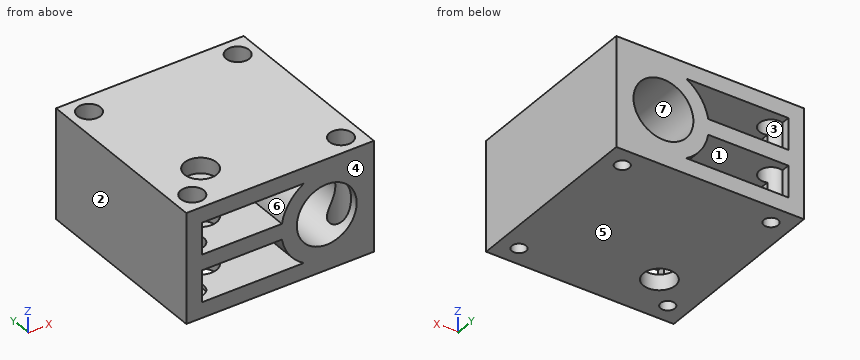
```python
from build123d import *

# Parameters (mm, degrees)
F2_W     = 48.25
F2_H     = 28.25
F2_R     = 7.7
F3_DEPTH = 24.2
F5_R     = 2.975
F6_DEPTH = 25.25
F4_R     = 1.825
F7_DEPTH = 28.25
F4_R_2   = 4.125
F8_DEPTH = 28.25


# Not quite as in the source:
# - a feature names something its author has since deleted; it is built from what else it names


with BuildPart() as f3:
    # F2 (on Front) → F3 (new body, symmetric)
    with BuildSketch(Plane.XZ):
        Rectangle(F2_W, F2_H)
        with BuildLine():
            ThreePointArc((23.5277925033, 2), (23.6568686252, 1.0037000824), (23.7, 0))
            ThreePointArc((23.7, 0), (23.6568686252, -1.0037000824), (23.5277925033, -2))
            ThreePointArc((23.5277925033, -2), (22.3372126342, -5.4801491728), (20.125, -8.4186920005))
            Line((20.125, -8.4186920005), (20.125, -10.125))
            Line((20.125, -10.125), (17.8629663994, -10.125))
            ThreePointArc((17.8629663994, -10.125), (15.9935594213, -10.9973398215), (14, -11.5277925033))
            ThreePointArc((14, -11.5277925033), (12, -11.7), (10, -11.5277925033))
            ThreePointArc((10, -11.5277925033), (8.0064405787, -10.9973398215), (6.1370336006, -10.125))
            Line((6.1370336006, -10.125), (-20.125, -10.125))
            Line((-20.125, -10.125), (-20.125, -2))
            Line((-20.125, -2), (-20.125, 2))
            Line((-20.125, 2), (-20.125, 10.125))
            Line((-20.125, 10.125), (6.1370336006, 10.125))
            ThreePointArc((6.1370336006, 10.125), (8.0064405787, 10.9973398215), (10, 11.5277925033))
            ThreePointArc((10, 11.5277925033), (12, 11.7), (14, 11.5277925033))
            ThreePointArc((14, 11.5277925033), (15.9935594213, 10.9973398215), (17.8629663994, 10.125))
            Line((17.8629663994, 10.125), (20.125, 10.125))
            Line((20.125, 10.125), (20.125, 8.4186920005))
            ThreePointArc((20.125, 8.4186920005), (22.3372126342, 5.4801491728), (23.5277925033, 2))
        make_face(mode=Mode.SUBTRACT)
        with BuildLine():
            Line((14, 10.125), (14, 11.5277925033))
            ThreePointArc((14, 11.5277925033), (12, 11.7), (10, 11.5277925033))
            Line((10, 11.5277925033), (10, 10.125))
            Line((10, 10.125), (14, 10.125))
        make_face()
        with BuildLine():
            Line((20.125, 2), (20.125, 8.4186920005))
            ThreePointArc((20.125, 8.4186920005), (19.045826619, 9.3405742466), (17.8629663994, 10.125))
            Line((17.8629663994, 10.125), (14, 10.125))
            Line((14, 10.125), (10, 10.125))
            Line((10, 10.125), (6.1370336006, 10.125))
            ThreePointArc((6.1370336006, 10.125), (2.4024206149, 6.6915222444), (0.4722074967, 2))
            ThreePointArc((0.4722074967, 2), (0.3, 0), (0.4722074967, -2))
            ThreePointArc((0.4722074967, -2), (2.4024206149, -6.6915222444), (6.1370336006, -10.125))
            Line((6.1370336006, -10.125), (10, -10.125))
            Line((10, -10.125), (14, -10.125))
            Line((14, -10.125), (17.8629663994, -10.125))
            ThreePointArc((17.8629663994, -10.125), (19.045826619, -9.3405742466), (20.125, -8.4186920005))
            Line((20.125, -8.4186920005), (20.125, -2))
            Line((20.125, -2), (20.125, 2))
        make_face()
        with Locations((12, 0)):
            Circle(F2_R, mode=Mode.SUBTRACT)
        with BuildLine():
            ThreePointArc((10, -11.5277925033), (12, -11.7), (14, -11.5277925033))
            Line((14, -11.5277925033), (14, -10.125))
            Line((14, -10.125), (10, -10.125))
            Line((10, -10.125), (10, -11.5277925033))
        make_face()
        with BuildLine():
            ThreePointArc((0.4722074967, -2), (0.3, 0), (0.4722074967, 2))
            Line((0.4722074967, 2), (-20.125, 2))
            Line((-20.125, 2), (-20.125, -2))
            Line((-20.125, -2), (0.4722074967, -2))
        make_face()
        with BuildLine():
            ThreePointArc((23.5277925033, -2), (23.6568686252, -1.0037000824), (23.7, 0))
            ThreePointArc((23.7, 0), (23.6568686252, 1.0037000824), (23.5277925033, 2))
            Line((23.5277925033, 2), (20.125, 2))
            Line((20.125, 2), (20.125, -2))
            Line((20.125, -2), (23.5277925033, -2))
        make_face()
        with BuildLine():
            Line((20.125, 2), (23.5277925033, 2))
            ThreePointArc((23.5277925033, 2), (22.3372126342, 5.4801491728), (20.125, 8.4186920005))
            Line((20.125, 8.4186920005), (20.125, 2))
        make_face()
        with BuildLine():
            ThreePointArc((20.125, -8.4186920005), (22.3372126342, -5.4801491728), (23.5277925033, -2))
            Line((23.5277925033, -2), (20.125, -2))
            Line((20.125, -2), (20.125, -8.4186920005))
        make_face()
        with BuildLine():
            Line((14, 10.125), (17.8629663994, 10.125))
            ThreePointArc((17.8629663994, 10.125), (15.9935594213, 10.9973398215), (14, 11.5277925033))
            Line((14, 11.5277925033), (14, 10.125))
        make_face()
        with BuildLine():
            Line((10, 10.125), (10, 11.5277925033))
            ThreePointArc((10, 11.5277925033), (8.0064405787, 10.9973398215), (6.1370336006, 10.125))
            Line((6.1370336006, 10.125), (10, 10.125))
        make_face()
        with BuildLine():
            ThreePointArc((14, -11.5277925033), (15.9935594213, -10.9973398215), (17.8629663994, -10.125))
            Line((17.8629663994, -10.125), (14, -10.125))
            Line((14, -10.125), (14, -11.5277925033))
        make_face()
        with BuildLine():
            ThreePointArc((6.1370336006, -10.125), (8.0064405787, -10.9973398215), (10, -11.5277925033))
            Line((10, -11.5277925033), (10, -10.125))
            Line((10, -10.125), (6.1370336006, -10.125))
        make_face()
        with BuildLine():
            ThreePointArc((17.8629663994, 10.125), (19.045826619, 9.3405742466), (20.125, 8.4186920005))
            Line((20.125, 8.4186920005), (20.125, 10.125))
            Line((20.125, 10.125), (17.8629663994, 10.125))
        make_face()
        with BuildLine():
            Line((20.125, -10.125), (20.125, -8.4186920005))
            ThreePointArc((20.125, -8.4186920005), (19.045826619, -9.3405742466), (17.8629663994, -10.125))
            Line((17.8629663994, -10.125), (20.125, -10.125))
        make_face()
    extrude(amount=F3_DEPTH, both=True)

    # F5 (on face) → F6 (cut)
    with BuildSketch(Plane.XY.offset(14.125)):
        with Locations((-19.125, 19.2)):
            Circle(F5_R)
        with Locations((19.125, -19.2)):
            Circle(F5_R)
        with Locations((-19.125, -19.2)):
            Circle(F5_R)
        with Locations((19.125, 19.2)):
            Circle(F5_R)
    extrude(amount=-F6_DEPTH, mode=Mode.SUBTRACT)

    # F4 (on face) → F7 (cut)
    with BuildSketch(Plane(origin=(0, 0, -14.125), x_dir=(1, 0, 0), z_dir=(0, 0, -1))):
        with Locations((-19.125, 19.2)):
            Circle(F4_R)
        with Locations((19.125, 19.2)):
            Circle(F4_R)
        with Locations((19.125, -19.2)):
            Circle(F4_R)
        with Locations((-19.125, -19.2)):
            Circle(F4_R)
    extrude(amount=-F7_DEPTH, mode=Mode.SUBTRACT)

    # F4 (on face) → F8 (cut)
    with BuildSketch(Plane(origin=(0, 0, -14.125), x_dir=(1, 0, 0), z_dir=(0, 0, -1))):
        with Locations((-12, 12)):
            Circle(F4_R_2)
    extrude(amount=-F8_DEPTH, mode=Mode.SUBTRACT)


solid = f3.part
```
Read the model definition and answer for the solid it produces. Units are mm, in the model's axes. Face numbers are marked on the shaded views. A direction names the side the tool comes from. Coordinates: 2 decimals unless noted, no trailing zeros. Loops run counter-clockwise (first coordinate to the right, second up) from the corner with the lowest first, then second, coordinate; pieces in that order, holes last. Notation, with made-up numbers: (58.25, -34.5) -> (100.25, -34.5) arc R20 ccw to (100.25, -4.5) -> close; hole circle Ø3 at (19, 53). An arc over 180 degrees is marked (long way). Return JSON: item names as keys, results as strings.
Item 1: Find section B-B (x = 12). Determine the outline of the cut face in (y, z) (3 decimals), plus the area to 3 significant figures.
Answers:
{"outline": "(-24.2, -14.125) -> (24.2, -14.125) -> (24.2, -7.7) -> (-24.2, -7.7) -> close; (-24.2, 7.7) -> (24.2, 7.7) -> (24.2, 14.125) -> (-24.2, 14.125) -> close", "area": "622 mm2"}
Item 2: Find section C-C (y = -6.5). Determine the outline of the cut face in (x, z) (3 decimals), plus the area to 3 significant figures.
Answers:
{"outline": "(-24.125, -14.125) -> (24.125, -14.125) -> (24.125, 14.125) -> (-24.125, 14.125) -> close; hole (-20.125, -10.125) -> (6.137, -10.125) arc R11.7 cw to (0.472, -2) -> (-20.125, -2) -> close; hole (-20.125, 2) -> (0.472, 2) arc R11.7 cw to (6.137, 10.125) -> (-20.125, 10.125) -> close; hole circle Ø15.4 at (12, 0)", "area": "811 mm2"}
Item 3: For a pull along Z with two mould halves and no side action, classify the marked faces 4, 5, 6 and 7 as +Z half, -Z half, draft (parallel to the pull), parting line (faces both ways), or undercut.
Answers:
{"face 4": "draft", "face 5": "-Z half", "face 6": "undercut", "face 7": "undercut"}
Item 4: A flat-ended cylindrical pin translates along its axis: P1, Ø3, axis at x = -19.5, y = 19, coming from the +Z side (3 decimals). Find the tip coordinate at first contact, or state that the pin passes through.
Answers:
{"P1": "stops at z = -11.125"}
Item 5: Find section D-D (z = 6.75). Determine the outline of the cut face in (x, y) (3 decimals).
Answers:
{"outline": "(-24.125, -24.2) -> (-20.125, -24.2) -> (-20.125, -22.002) arc R2.975 cw to (-20.125, -16.398) -> (-20.125, 16.398) arc R2.975 cw to (-20.125, 22.002) -> (-20.125, 24.2) -> (-24.125, 24.2) -> close; (2.443, -24.2) -> (8.295, -24.2) -> (8.295, 24.2) -> (2.443, 24.2) -> close; (15.705, -24.2) -> (24.125, -24.2) -> (24.125, 24.2) -> (15.705, 24.2) -> close; hole circle Ø5.95 at (19.125, -19.2); hole circle Ø5.95 at (19.125, 19.2)"}
Item 6: Find the intervals of material crossed by probe 1 along Z at (x, y) = (0, 13.5) (3 decimals); probe 2 along X at (y, z) = (-12, -11.35) (3 decimals); probe 3 along X at (y, z) = (-1.5, -5.5) (3 decimals), in increasing order.
Answers:
{"probe 1": "z = -14.125 to -10.125, -2 to 2, 10.125 to 14.125", "probe 2": "x = -24.125 to -16.125, -7.875 to 24.125", "probe 3": "x = -24.125 to -20.125, 1.673 to 6.611, 17.389 to 24.125"}
Item 7: Find section A-A (y = -12). Determine the outline of the cut face in (x, z) (3 decimals), plus the area to 3 significant figures.
Answers:
{"outline": "(-24.125, -14.125) -> (-16.125, -14.125) -> (-16.125, -10.125) -> (-20.125, -10.125) -> (-20.125, -2) -> (-16.125, -2) -> (-16.125, 2) -> (-20.125, 2) -> (-20.125, 10.125) -> (-16.125, 10.125) -> (-16.125, 14.125) -> (-24.125, 14.125) -> close; (-7.875, -14.125) -> (24.125, -14.125) -> (24.125, 14.125) -> (-7.875, 14.125) -> (-7.875, 10.125) -> (6.137, 10.125) arc R11.7 ccw to (0.472, 2) -> (-7.875, 2) -> (-7.875, -2) -> (0.472, -2) arc R11.7 ccw to (6.137, -10.125) -> (-7.875, -10.125) -> close; hole circle Ø15.4 at (12, 0)", "area": "712 mm2"}
Item 8: For the marked faces 1, 2 and 3, determine the directions among +Z, -Z, +X, -X, +Y, -Y from which every point of the face is accessible in a straight line to the end or side of a thin tool.
Answers:
{"face 1": "+Y, -Y", "face 2": "+Z, -Z, -X, +Y, -Y", "face 3": "+Z"}
